from build123d import *

# Parameters (mm, degrees)
F1_W      = 9
F1_H      = 83
F2_DEPTH  = 63
F3_R      = 2.85
F4_DEPTH  = 3.5
F5_R      = 1.6
F6_DEPTH  = 25
F7_W      = 40
F7_H      = 10
F8_DEPTH  = 20.2
F9_W      = 4.8
F9_H      = 40
F10_DEPTH = 2
F11_SIZE  = 1.8
F12_R     = 1.6
F13_DEPTH = 25
F14_W     = 4.8
F14_H     = 40
F15_DEPTH = 2
F16_SIZE  = 1.8
F17_R     = 1.6
F18_DEPTH = 25
F19_R     = 2.85
F20_DEPTH = 3.5
F21_R     = 2.85
F22_DEPTH = 3.5
F23_R     = 1.5
F24_DEPTH = 10


with BuildPart() as f2:
    # F1 (on Top) → F2 (new body)
    with BuildSketch(Plane.XY):
        with Locations((4.5, 41.5)):
            Rectangle(F1_W, F1_H)
    extrude(amount=F2_DEPTH)

    # F3 (on face) → F4 (cut)
    with BuildSketch(Plane.YZ.offset(9)):
        with Locations((8.5, 40.5)):
            Circle(F3_R)
        with Locations((8.5, 22.5)):
            Circle(F3_R)
        with Locations((76.5, 56.5)):
            Circle(F3_R)
        with Locations((76.5, 38.5)):
            Circle(F3_R)
        with Locations((76.5, 24.5)):
            Circle(F3_R)
        with Locations((76.5, 6.5)):
            Circle(F3_R)
    extrude(amount=-F4_DEPTH, mode=Mode.SUBTRACT)

    # F5 (on face) → F6 (cut)
    with BuildSketch(Plane.YZ.offset(9)):
        with Locations((8.5, 40.5)):
            Circle(F5_R)
        with Locations((8.5, 22.5)):
            Circle(F5_R)
        with Locations((76.5, 24.5)):
            Circle(F5_R)
        with Locations((76.5, 38.5)):
            Circle(F5_R)
        with Locations((76.5, 56.5)):
            Circle(F5_R)
        with Locations((76.5, 6.5)):
            Circle(F5_R)
    extrude(amount=-F6_DEPTH, mode=Mode.SUBTRACT)

    # F7 (on face) → F8 (join)
    with BuildSketch(Plane.YZ.offset(9)):
        with Locations((43, 16.4)):
            Rectangle(F7_W, F7_H)
        with Locations((43, 46.6)):
            Rectangle(F7_W, F7_H)
    extrude(amount=F8_DEPTH)

    # F9 (on face) → F10 (join)
    with BuildSketch(Plane(origin=(0, 0, 41.6), x_dir=(1, 0, 0), z_dir=(0, 0, -1))):
        with Locations((19.1, -43)):
            Rectangle(F9_W, F9_H)
    extrude(amount=F10_DEPTH)

    # F11
    f11_edges = [f2.edges().sort_by_distance(p)[0] for p in [
        (21.5, 43, 39.6),
        (16.7, 43, 39.6),
    ]]
    chamfer(f11_edges, length=F11_SIZE)

    # F12 (on face) → F13 (cut)
    with BuildSketch(Plane(origin=(0, 0, 39.6), x_dir=(1, 0, 0), z_dir=(0, 0, -1))):
        with Locations((19.1, -33)):
            Circle(F12_R)
        with Locations((19.1, -53)):
            Circle(F12_R)
    extrude(amount=-F13_DEPTH, mode=Mode.SUBTRACT)

    # F14 (on face) → F15 (join)
    with BuildSketch(Plane.XY.offset(21.4)):
        with Locations((19.1, 43)):
            Rectangle(F14_W, F14_H)
    extrude(amount=F15_DEPTH)

    # F16
    f16_edges = [f2.edges().sort_by_distance(p)[0] for p in [
        (21.5, 43, 23.4),
        (16.7, 43, 23.4),
    ]]
    chamfer(f16_edges, length=F16_SIZE)

    # F17 (on face) → F18 (cut)
    with BuildSketch(Plane.XY.offset(23.4)):
        with Locations((19.1, 33)):
            Circle(F17_R)
        with Locations((19.1, 53)):
            Circle(F17_R)
    extrude(amount=-F18_DEPTH, mode=Mode.SUBTRACT)

    # F19 (on face) → F20 (cut)
    with BuildSketch(Plane(origin=(0, 0, 11.4), x_dir=(1, 0, 0), z_dir=(0, 0, -1))):
        with Locations((19.1, -33)):
            Circle(F19_R)
        with Locations((19.1, -53)):
            Circle(F19_R)
    extrude(amount=-F20_DEPTH, mode=Mode.SUBTRACT)

    # F21 (on face) → F22 (cut)
    with BuildSketch(Plane.XY.offset(51.6)):
        with Locations((19.1, 53)):
            Circle(F21_R)
        with Locations((19.1, 33)):
            Circle(F21_R)
    extrude(amount=-F22_DEPTH, mode=Mode.SUBTRACT)

    # F23 (on face) → F24 (cut)
    with BuildSketch(Plane.YZ.offset(29.2)):
        with Locations((56.5, 16.4)):
            Circle(F23_R)
        with Locations((29.5, 16.4)):
            Circle(F23_R)
        with Locations((29.5, 46.6)):
            Circle(F23_R)
        with Locations((56.5, 46.6)):
            Circle(F23_R)
    extrude(amount=-F24_DEPTH, mode=Mode.SUBTRACT)


solid = f2.part
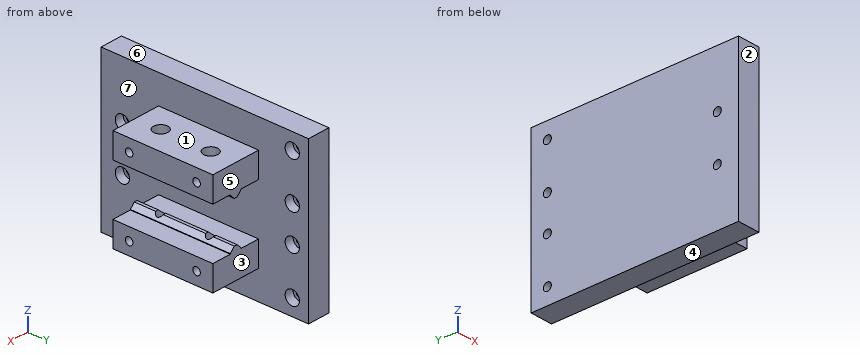
Work out the finished part from the listing and answer in its coordinate system (mm). Face numbers are marked on the shaded views. A direction names the side the tool comes from. Coordinates: 2 decimals unless noted, no trailing zeros. Write each loop counter-clockwise with the first axis right and the second up, starting at its lowest first coordinate (ties: lowest second). Pieces come first, ordered by that corner, then holes. Notation, with made-up numbers: M 66,70.25 L 98,70.25 A20 ccw 98,105.25 Z; hole C 2.25,21 d7. An arc over 180 degrees is marked long. Answer as CSV lines item,"result". Start each with the question number.
Item 1: Section C-C on y = 47.5 is taken. Write down the section's boundary in (x, z).
Item 2: Flat-ended cylindrical pins translate along their axes: P1, Ø13, axis at x = 18, z = 20.5, coming from the +Y side; P2, Ø5, axis at y = 76.5, z = 6.5, coming from the +X side; P3, Ø1.3, axis at x = 19, y = 29, coming from the +Z side. Find the tip coordinate at first contact, or state that the pin passes through.
Item 3: A tool of negligible diameter and unlimited length cuts with its end or side. For the marked faces 1, 2 and 3, from which of +Z, -Z, +X, -X, +Y, -Y can it reach the whole face along a straight path? Write none if from no direction.
Item 4: Section D-D on z = 16.4 is taken. Write down the section's boundary in (x, y), and give its area (3 significant figures).
Item 5: Section B-B on y = 8.5 is taken. Write down the section's boundary in (x, z), and give its area (3 significant figures).
Item 6: Determine the mould class of the marked faces 4, 5, 6 and 7 for opening direction Z: released by +Z, released by -Z, zero draft, split by the parting line, or undercut.
Item 7: Consider L1, parallel to Z at x = 26.25, y = 29.5; L2, parallel to Z at x = 3.9, y = 76.5; L3, parallel to Y at x = 19.1, z = 49.7. Determine where each line is inside the solid, lowest interval first.
Item 8: Section A-A on z = 6.5 is taken. Write down the section's boundary in (x, y), and give its area (3 significant figures).
Checks:
1,outline,"M 0,0 L 9,0 L 9,11.4 L 29.2,11.4 L 29.2,21.4 L 21.5,21.4 L 21.5,21.6 L 19.7,23.4 L 18.5,23.4 L 16.7,21.6 L 16.7,21.4 L 9,21.4 L 9,41.6 L 16.7,41.6 L 16.7,41.4 L 18.5,39.6 L 19.7,39.6 L 21.5,41.4 L 21.5,41.6 L 29.2,41.6 L 29.2,51.6 L 9,51.6 L 9,63 L 0,63 Z"
2,P1,"stops at y = 63"
2,P2,"stops at x = 5.5"
2,P3,"stops at z = 51.6"
3,face 1,"+Z, +X, +Y, -Y"
3,face 2,"+Z, -Z, +X, -X, -Y"
3,face 3,"+Z, -Z, +X, +Y"
4,outline,"M 0,0 L 9,0 L 9,23 L 29.2,23 L 29.2,28 L 19.2,28 L 19.2,31 L 29.2,31 L 29.2,55 L 19.2,55 L 19.2,58 L 29.2,58 L 29.2,63 L 9,63 L 9,83 L 0,83 Z; hole C 19.1,33 d3.2; hole C 19.1,53 d3.2"
4,area,"1,480 mm²"
5,outline,"M 0,0 L 9,0 L 9,19.65 L 5.5,19.65 L 5.5,20.9 L 0,20.9 Z; M 0,24.1 L 5.5,24.1 L 5.5,25.35 L 9,25.35 L 9,37.65 L 5.5,37.65 L 5.5,38.9 L 0,38.9 Z; M 0,42.1 L 5.5,42.1 L 5.5,43.35 L 9,43.35 L 9,63 L 0,63 Z"
5,area,"492 mm²"
6,face 4,"released by -Z"
6,face 5,"zero draft"
6,face 6,"released by +Z"
6,face 7,"undercut"
7,L1,"z = 11.4 to 14.9, 17.9 to 21.4, 41.6 to 45.1, 48.1 to 51.6"
7,L2,"z = 0 to 4.9, 8.1 to 22.9, 26.1 to 36.9, 40.1 to 54.9, 58.1 to 63"
7,L3,"y = 23 to 30.15, 35.85 to 50.15, 55.85 to 63"
8,outline,"M 0,0 L 9,0 L 9,73.65 L 5.5,73.65 L 5.5,74.9 L 0,74.9 Z; M 0,78.1 L 5.5,78.1 L 5.5,79.35 L 9,79.35 L 9,83 L 0,83 Z"
8,area,"709 mm²"
